CAD build for the part. Positions are in the model's coordinates, mm. Face numbers are marked on the shaded views. A direction names the side the tool comes from. Give positions to 0.01 mm unless a question says otherwise; leave off trailing zeros. Order: outer loops, then holes, each group sorted by start corner. A loop starts at its lowest first (then second) coordinate and runs counter-clockwise, first axis right, second up.
Item 1: Band-saw the part on C-C on x = -10.5. Give the cut face in (y, z) (3 decimals).
Item 2: Band-saw the part on D-D on z = 31.5. Give the cut face in (x, y), plus the area to 3 significant figures.
Item 3: Wall check: L1, parallel to Y at x = 46.5, z = 26; L2, parallel to X at y = 10, z = 12.5. Give the ranges that are in metal, low to high.
Item 4: Band-saw the part on A-A on y = 28.5. Give the cut face in (x, z) (3 decimals).
Item 5: Which spindle directions (+Z, -Z, +X, -X, +Y, -Y) get a long thin tool onto all of the face, cutting with end or side? Do the marked faces 1 and 2. Say none if no direction does.
Item 6: Flat gauge pins, fed straight in: P1, Ø8.5, axis at x = 33.98, z = 20.64, coming from the +Y side; P2, Ø12, axis at x = -11, z = 5.5, coming from the +Y side; P3, Ø12.5, axis at y = 62, z = 19.5, coming from the +X side. Where does each tip first touch, or does it go through?
Item 7: Band-saw the part on B-B on z = 22.5. Give the cut face in (x, y).
```python
from build123d import *

# Parameters (mm, degrees)
BOSS_EXTRUDE1_DEPTH = 41.275
SKETCH2_R           = 7.14375
CUT_EXTRUDE1_DEPTH  = 41.275
SKETCH3_R           = 7.14375
CUT_EXTRUDE2_DEPTH  = 41.275


with BuildPart() as part:
    # Sketch1 → Boss-Extrude1 (new body)
    with BuildSketch(Plane.XY):
        with BuildLine():
            Line((-35.867305165, 89.962083988), (-42.217305165, 89.962083988))
            Line((-42.217305165, 89.962083988), (-42.217305165, -2.112916012))
            Line((-42.217305165, -2.112916012), (-42.217305165, -5.922916012))
            ThreePointArc((-42.217305165, -5.922916012), (-41.473356389, -7.718967236), (-39.677305165, -8.462916012))
            Line((-39.677305165, -8.462916012), (-35.867305165, -8.462916012))
            Line((-35.867305165, -8.462916012), (53.032694835, -8.462916012))
            Line((53.032694835, -8.462916012), (53.032694835, -2.112916012))
            Line((53.032694835, -2.112916012), (-33.327305165, -2.112916012))
            ThreePointArc((-33.327305165, -2.112916012), (-35.123356389, -1.368967236), (-35.867305165, 0.427083988))
            Line((-35.867305165, 0.427083988), (-35.867305165, 89.962083988))
        make_face()
    extrude(amount=BOSS_EXTRUDE1_DEPTH)

    # Sketch2 → Cut-Extrude1 (cut)
    with BuildSketch(Plane(origin=(-35.867305165, 0, 0), x_dir=(0, 0, -1), z_dir=(1, 0, 0))):
        with Locations(Location((-20.6375, 70.912083988, 0), (0, 0, 90))):
            Circle(SKETCH2_R)
        with Locations(Location((-20.6375, 23.287083988, 0), (0, 0, 90))):
            Circle(SKETCH2_R)
    extrude(amount=-CUT_EXTRUDE1_DEPTH, mode=Mode.SUBTRACT)

    # Sketch3 → Cut-Extrude2 (cut)
    with BuildSketch(Plane(origin=(0, -2.112916012, 0), x_dir=(1, 0, 0), z_dir=(0, 1, 0))):
        with Locations(Location((-13.769305165, -20.6375, 0), (0, 0, 180))):
            Circle(SKETCH3_R)
        with Locations(Location((33.982694835, -20.6375, 0), (0, 0, 180))):
            Circle(SKETCH3_R)
    extrude(amount=-CUT_EXTRUDE2_DEPTH, mode=Mode.SUBTRACT)


solid = part.part
```
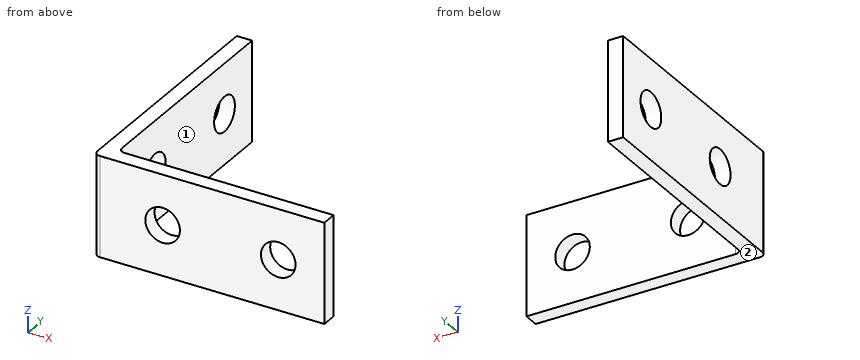
The answers:
1. outline: (-8.463, 0) - (-2.113, 0) - (-2.113, 14.286) - (-8.463, 14.286) - close; (-8.463, 26.989) - (-2.113, 26.989) - (-2.113, 41.275) - (-8.463, 41.275) - close
2. outline: (-42.22, -5.92) arc R2.54 ccw to (-39.68, -8.46) - (53.03, -8.46) - (53.03, -2.11) - (-33.33, -2.11) arc R2.54 cw to (-35.87, 0.43) - (-35.87, 89.96) - (-42.22, 89.96) - close
2. area: 1,190 mm2
3. L1: y = -8.46 to -2.11
3. L2: x = -42.22 to -35.87
4. outline: (-42.217, 0) - (-35.867, 0) - (-35.867, 15.753) - (-42.217, 15.753) - close; (-42.217, 25.522) - (-35.867, 25.522) - (-35.867, 41.275) - (-42.217, 41.275) - close
5. face 1: +Z, -Z, +X, +Y
5. face 2: -Z, +X, -X, +Y, -Y
6. P1: passes through
6. P2: stops at y = -2.11
6. P3: stops at x = -35.87
7. outline: (-42.22, -5.92) arc R2.54 ccw to (-39.68, -8.46) - (-20.67, -8.46) - (-20.67, -2.11) - (-33.33, -2.11) arc R2.54 cw to (-35.87, 0.43) - (-35.87, 16.39) - (-42.22, 16.39) - close; (-42.22, 30.18) - (-35.87, 30.18) - (-35.87, 64.02) - (-42.22, 64.02) - close; (-42.22, 77.81) - (-35.87, 77.81) - (-35.87, 89.96) - (-42.22, 89.96) - close; (-6.87, -8.46) - (27.09, -8.46) - (27.09, -2.11) - (-6.87, -2.11) - close; (40.88, -8.46) - (53.03, -8.46) - (53.03, -2.11) - (40.88, -2.11) - close
